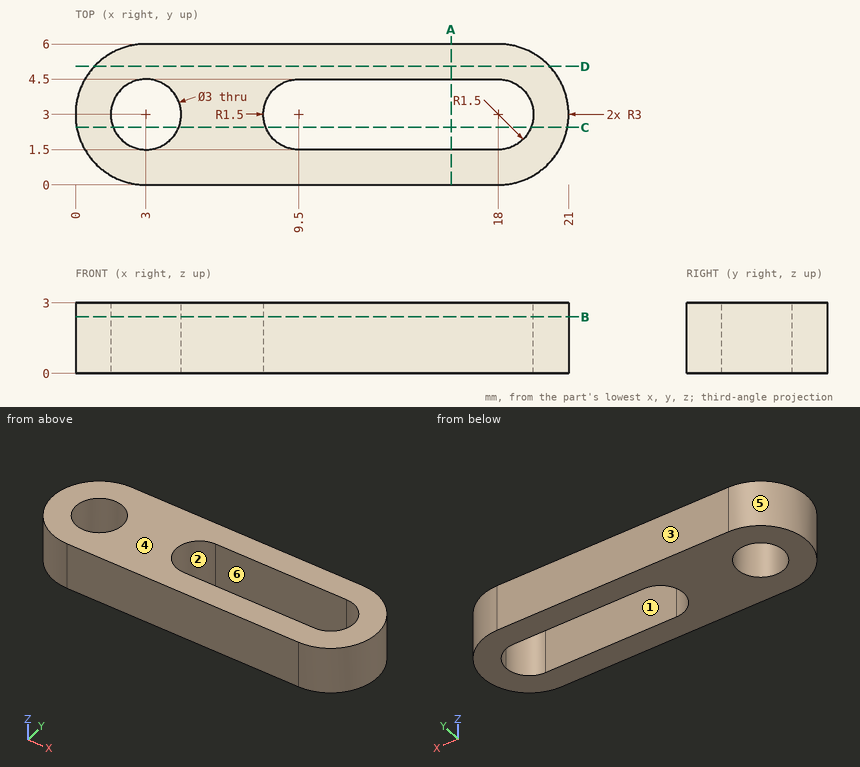
Input: dimensioned drawing with shaded views. Units: mm. Origin: part minimum x, y, z. A direction names the side the tool comes from. Give positions to 0.01 mm unless a question says otherwise; leave off trailing zeros. Write each loop counter-clockwise with the first axis right and the second up, starting at its lowest first coordinate (ties: lowest second). Pieces come first, ordered by that corner, then holes. Notation, with made-up numbers: (65.25, 13) -> (115.25, 13) arc R21 ccw to (115.25, 47) -> close; hole circle Ø6 at (-1, 56.5). An arc over 180 degrees is marked (long way). Return JSON: item names as keys, results as strings. Group by question number.
1. Section B-B, the plane z = 2.4. Output: boundary loops of the cut face in (x, y), then the cut area to 3 significant figures.
2. Section C-C, the plane y = 2.45. Output: boundary loops of the cut face in (x, z).
3. Pin query (flat end, axial travel): pin 1 Ø1 at (y, z) = (2, 2) entering from +X; pin 2 Ø1.8 at (x, y) = (3, 3) entering from +Z; pin 3 Ø3 at (x, y) = (16, 2) entering from +Z. Return the tip coordinate at first contact, or that it passes through.
4. Section D-D, the plane y = 5.05. Output: boundary loops of the cut face in (x, z).
5. Material intervals for line 1 (Y direction, x = 3, z = 1.15); line 2 (X direction, y = 2.7, z = 1.95); line 3 (X direction, y = 2.6, z = 2.8), sorted ascending. Write a range as from..to.
6. Section A-A, the plane x = 16. Output: boundary loops of the cut face in (y, z), then the cut area to 3 significant figures.
7. Mould query, pull axis Y, two halves, no side actions, for the marked faces 1, 2, 3 and 4. Classes: +Y half, -Y half, draft (parallel to the pull), parting line (faces both ways), or undercut.
8. Access query for the marked faces 5 and 6. Directions: +Z, -Z, +X, -X, +Y, -Y. A direction counts if a zero-diameter tool reaches every point of the face in a straight line with its end or side. Return the directions, or none.
Determined:
{
 "1": {"outline": "(3, 0) -> (18, 0) arc R3 ccw to (18, 6) -> (3, 6) arc R3 ccw to start; hole circle Ø3 at (3, 3); hole (9.5, 1.5) -> (18, 1.5) arc R1.5 ccw to (19.5, 3) arc R1.5 ccw to (18, 4.5) -> (9.5, 4.5) arc R1.5 ccw to start", "area": "78.6 mm2"},
 "2": {"outline": "(0.05, 0) -> (1.6, 0) -> (1.6, 3) -> (0.05, 3) -> close; (4.4, 0) -> (8.1, 0) -> (8.1, 3) -> (4.4, 3) -> close; (19.4, 0) -> (20.95, 0) -> (20.95, 3) -> (19.4, 3) -> close"},
 "3": {"pin 1": "stops at x = 20.96", "pin 2": "passes through", "pin 3": "stops at z = 3"},
 "4": {"outline": "(0.81, 0) -> (20.19, 0) -> (20.19, 3) -> (0.81, 3) -> close"},
 "5": {"line 1": "y = 0..1.5, 4.5..6", "line 2": "x = 0.02..1.53, 4.47..8.03, 19.47..20.98", "line 3": "x = 0.03..1.55, 4.45..8.05, 19.45..20.97"},
 "6": {"outline": "(0, 0) -> (1.5, 0) -> (1.5, 3) -> (0, 3) -> close; (4.5, 0) -> (6, 0) -> (6, 3) -> (4.5, 3) -> close", "area": "9.00 mm2"},
 "7": {"face 1": "undercut", "face 2": "undercut", "face 3": "+Y half", "face 4": "draft"},
 "8": {"face 5": "+Z, -Z, -X", "face 6": "+Z, -Z"}
}
